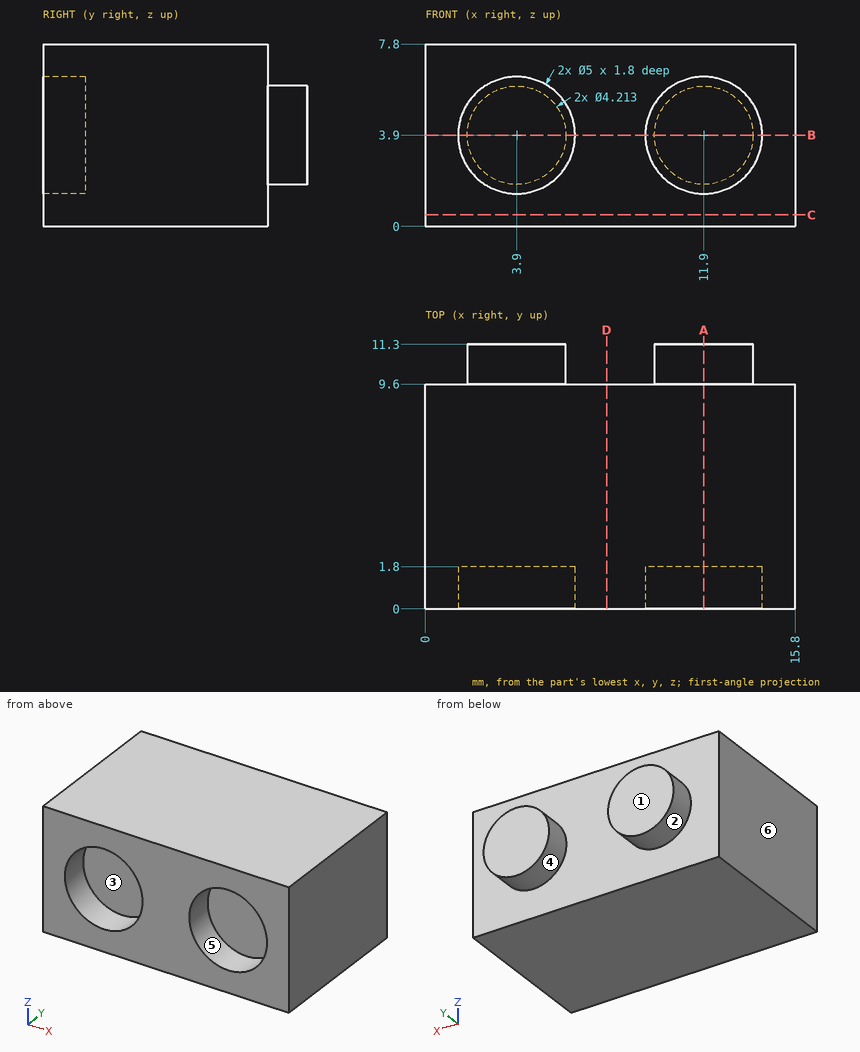
For this review, use the dimensioned drawing (mm, ordinates from the lowest corner) and the shaded views. A direction names the side the tool comes from. Round coordinates to 2 decimals unless told otherwise and drop trailing zeros. Write each loop counter-clockwise with the first axis right and the second up, starting at its lowest first coordinate (ties: lowest second). Pieces come first, ordered by that corner, then holes. Notation, with made-up numbers: M 85.25,55 L 98.25,55 A12 ccw 98.25,78 Z; hole C -6,-24.75 d7. An arc over 180 degrees is marked long. Answer as CSV lines item,"result". Start each with the question number.
Q1. The part is to be moulded in two halves that separate along Z. For the marked faces 1, 2 and 3, say which applies: +Z half, -Z half, draft (parallel to the pull), parting line (faces both ways), or undercut.
Q2. Consider section D-D, the plane x = 7.75. Give the boundary of the cut face in (y, z), then the cut area to 3 significant figures.
Q3. Clearance check with a flat-ended pin moving along its axis: P1, Ø2.5, axis at x = 11.5, z = 4.5, coming from the -Y side. State where the tip first meets the part, or that it passes through.
Q4. Consider section B-B, the plane z = 3.9. Give the boundary of the cut face in (x, y).
Q5. Wall thickness on line 1 along X through (y, z) = (0.5, 5.25) (1 decimal); line 2 along Z through (x, y) = (3.9, 0.45); line 3 along Y through (x, z) = (3.5, 5.5): over which ranges is each line inside the solid? List them lowest first.
Q6. Tool access review of the marked faces 4, 5 and 6: name each direction out of +Z, -Z, +X, -X, +Y, -Y from which nothing blocks a thin tool from reaching the whole face with its end or side.
Q7. Consider section A-A, the plane x = 11.9. Give the boundary of the cut face in (y, z).
Q8. Consider section C-C, the plane z = 0.5. Give the boundary of the cut face in (x, y).
Result set:
1,face 1,"draft"
1,face 2,"parting line"
1,face 3,"undercut"
2,outline,"M 0,0 L 9.6,0 L 9.6,7.8 L 0,7.8 Z"
2,area,"74.9 mm²"
3,P1,"stops at y = 1.8"
4,outline,"M 0,0 L 1.4,0 L 1.4,1.8 L 6.4,1.8 L 6.4,0 L 9.4,0 L 9.4,1.8 L 14.4,1.8 L 14.4,0 L 15.8,0 L 15.8,9.6 L 14.01,9.6 L 14.01,11.3 L 9.79,11.3 L 9.79,9.6 L 6.01,9.6 L 6.01,11.3 L 1.79,11.3 L 1.79,9.6 L 0,9.6 Z"
5,line 1,"x = 0 to 1.8, 6 to 9.8, 14 to 15.8"
5,line 2,"z = 0 to 1.4, 6.4 to 7.8"
5,line 3,"y = 1.8 to 11.3"
6,face 4,"+Y"
6,face 5,"-Y"
6,face 6,"+Z, -Z, -X, +Y, -Y"
7,outline,"M 0,0 L 9.6,0 L 9.6,1.79 L 11.3,1.79 L 11.3,6.01 L 9.6,6.01 L 9.6,7.8 L 0,7.8 L 0,6.4 L 1.8,6.4 L 1.8,1.4 L 0,1.4 Z"
8,outline,"M 0,0 L 15.8,0 L 15.8,9.6 L 0,9.6 Z"
